Here's how the part is built. I have some questions about the finished solid (model axes, mm). A direction names the side the tool comes from. Coordinates: 2 decimals unless noted, no trailing zeros. Order: outer loops, then holes, each group sorted by start corner. A loop starts at its lowest first (then second) coordinate and runs counter-clockwise, first axis right, second up. Notation, with made-up numbers: (84.5, -3) - (117.5, -3) arc R19 ccw to (117.5, 25) - close; hole circle Ø10 at (4.5, 33.25). An arc over 180 degrees is marked (long way). Answer as CSV lines item,"result". Start each with the question number.
Q1. Suppose I cut it at D-D (x = -18). Please give me the cut outline in (y, z), then the cut area to 3 significant figures.
Q2. For faces 5 (the face through (-15, 0, 7)), 6 (the face through (-16, -5, 10)), 7 (the face through (-0.54, -2.44, 11.26)), 8 (the face through (-16, 5, -9)), which set-ups out of +Z, -Z, +X, -X, +Y, -Y let a thin tool reach every point of the face, with its end or its side?
Q3. Suppose I cut it at A-A (x = 1.5). Please give me the cut outline in (y, z), then the cut area to 3 significant figures.
Q4. Suppose I cut it at C-C (z = 0). Please give me the cut outline in (x, y).
Q5. For pin 1 Ø2.5 at (x, z) = (-16, -10.5) entering from -Y; pin 2 Ø2.5 at (x, z) = (-16.5, -9) entering from +Y; pin 3 Ø1 at (y, z) = (-3, -4) entering from -X; pin 4 Ø11.5 at (y, z) = (-0.5, -2.5) entering from -X, each with a flat end and sliding along its axis, tell me the tip position at first contact or that it passes through.
Q6. I need wall thicknesses on line 1 (Z direction, x = 3.5, y = -3); line 2 (Y direction, x = 9.5, z = -3); line 3 (X direction, y = 10.95, z = 0). Which ranges of each line are inside material? Lowest first, please.
Q7. Suppose I cut it at B-B (y = 0). Please give me the cut outline in (x, z), then the cut area to 4 significant figures.
Q8. Thinking about a two-plate mould opening in X: for faces 1 (the face through (-16, 5, 9)), 2 (the face through (-15.253, 0.121, -9.535)), 3 (the face through (-2.44, 11.01, -0.54)), 4 (the face through (-24, 0, -10)), which applies, released by +X, released by -X, zero draft, split by the parting line, or undercut?
from build123d import *

# Parameters (mm, degrees)
SKETCH1_W            = 24
SKETCH1_H            = 24
BOSS_EXTRUDE1_DEPTH  = 11.5
SKETCH2_W            = 21
SKETCH2_H            = 21
CUT_EXTRUDE1_DEPTH   = 21
SKETCH3_R            = 2.5
CUT_EXTRUDE2_DEPTH   = 3
SKETCH4_R            = 2.5
CUT_EXTRUDE3_DEPTH   = 3
BOSS_EXTRUDE3_DEPTH  = 12
SKETCH9_R            = 2.75
CUT_EXTRUDE5_DEPTH   = 5
FILLET2_R            = 3
FILLET2_OF_MIRROR1_R = 3


with BuildPart() as part:
    # Sketch1 → Boss-Extrude1 (new, symmetric)
    with BuildSketch(Plane(origin=(0, 0, 0), x_dir=(1, 0, 0), z_dir=(0, 1, 0))):
        Rectangle(SKETCH1_W, SKETCH1_H)
    extrude(amount=BOSS_EXTRUDE1_DEPTH, both=True)

    # Sketch2 → Cut-Extrude1 (cut)
    with BuildSketch(Plane(origin=(12, 0, 0), x_dir=(0, 0, -1), z_dir=(1, 0, 0))):
        Rectangle(SKETCH2_W, SKETCH2_H)
    extrude(amount=-CUT_EXTRUDE1_DEPTH, mode=Mode.SUBTRACT)

    # Sketch3 → Cut-Extrude2 (cut)
    with BuildSketch(Plane(origin=(0, 11.5, 0), x_dir=(1, 0, 0), z_dir=(0, 1, 0))):
        with Locations(Location((0, 0, 0), (0, 0, 270))):
            Circle(SKETCH3_R)
    extrude(amount=-CUT_EXTRUDE2_DEPTH, mode=Mode.SUBTRACT)

    # Sketch4 → Cut-Extrude3 (cut)
    with BuildSketch(Plane.XY.offset(12)):
        Circle(SKETCH4_R)
    extrude(amount=-CUT_EXTRUDE3_DEPTH, mode=Mode.SUBTRACT)

    # Sketch8 → Boss-Extrude3 (add)
    with BuildSketch(Plane.ZY.offset(12)):
        Polygon((-7, 0), (-7, 5), (-12, 5), (-12, 0), (-12, -5), (-7, -5), align=None)
    boss_extrude3 = extrude(amount=BOSS_EXTRUDE3_DEPTH)

    # Sketch9 → Cut-Extrude5 (cut)
    with BuildSketch(Plane(origin=(0, 0, -12), x_dir=(-1, 0, 0), z_dir=(0, 0, -1))):
        with Locations((18, 0)):
            Circle(SKETCH9_R)
    cut_extrude5 = extrude(amount=-CUT_EXTRUDE5_DEPTH, mode=Mode.SUBTRACT)

    # Fillet2
    fillet2_edges = [part.edges().sort_by_distance(p)[0] for p in [
        (-24, 5, -9.5),
        (-24, -5, -9.5),
    ]]
    fillet(fillet2_edges, radius=FILLET2_R)

    # Mirror1: Boss-Extrude3, Cut-Extrude5 across plane
    add(boss_extrude3.mirror(Plane.XY))
    add(cut_extrude5.mirror(Plane.XY), mode=Mode.SUBTRACT)

    # Fillet2 of Mirror1
    fillet2_of_mirror1_edges = [part.edges().sort_by_distance(p)[0] for p in [
        (-24, 5, 9.5),
        (-24, -5, 9.5),
    ]]
    fillet(fillet2_of_mirror1_edges, radius=FILLET2_OF_MIRROR1_R)


solid = part.part
Here are the results:
1,outline,"(-5, -12) - (-2.75, -12) - (-2.75, -7) - (-5, -7) - close; (-5, 7) - (-2.75, 7) - (-2.75, 12) - (-5, 12) - close; (2.75, -12) - (5, -12) - (5, -7) - (2.75, -7) - close; (2.75, 7) - (5, 7) - (5, 12) - (2.75, 12) - close"
1,area,"45.0 mm²"
2,face 5,"-X, +Y, -Y"
2,face 6,"+Z, -Z, -X, -Y"
2,face 7,"+Z"
2,face 8,"+Z, -Z, -X, +Y"
3,outline,"(-11.5, -12) - (11.5, -12) - (11.5, -2) - (10.5, -2) - (10.5, -10.5) - (-10.5, -10.5) - (-10.5, 10.5) - (-2, 10.5) - (-2, 12) - (-11.5, 12) - close; (2, 10.5) - (10.5, 10.5) - (10.5, 2) - (11.5, 2) - (11.5, 12) - (2, 12) - close"
3,area,"101 mm²"
4,outline,"(-12, -11.5) - (12, -11.5) - (12, -10.5) - (-9, -10.5) - (-9, 10.5) - (-2.5, 10.5) - (-2.5, 11.5) - (-12, 11.5) - close; (2.5, 10.5) - (12, 10.5) - (12, 11.5) - (2.5, 11.5) - close"
5,pin 1,"stops at y = -5"
5,pin 2,"stops at y = 5"
5,pin 3,"stops at x = -12"
5,pin 4,"stops at x = -24"
6,line 1,"z = -12 to -10.5, 10.5 to 12"
6,line 2,"y = -11.5 to -10.5, 10.5 to 11.5"
6,line 3,"x = -12 to -2.5, 2.5 to 12"
7,outline,"(-24, -12) - (-20.75, -12) - (-20.75, -7) - (-24, -7) - close; (-24, 7) - (-20.75, 7) - (-20.75, 12) - (-24, 12) - close; (-15.25, -12) - (12, -12) - (12, -10.5) - (-9, -10.5) - (-9, 10.5) - (-2.5, 10.5) - (-2.5, 12) - (-15.25, 12) - (-15.25, 7) - (-12, 7) - (-12, -7) - (-15.25, -7) - close; (2.5, 10.5) - (12, 10.5) - (12, 12) - (2.5, 12) - close"
7,area,"192.5 mm²"
8,face 1,"zero draft"
8,face 2,"undercut"
8,face 3,"undercut"
8,face 4,"released by -X"
